Work out the finished part from the listing and answer in its coordinate system (mm). A direction names the side the tool comes from. Round coordinates to 2 decimals unless told otherwise and drop trailing zeros. Write each loop counter-clockwise with the first axis right and the second up, starting at its lowest first coordinate (ties: lowest second). Pieces come first, ordered by that corner, then holes.
1. Determine the mould class of faces 1 (the face through (-5.615, -25.284, 37.567)), 2 (the face through (3.175, 18, 32)), 3 (the face through (6.487, -20.284, 59.719)), 4 (the face through (0, -17, 0)) for opening direction X: pulls with the +X half, pulls with the -X half, needs draft (parallel to the pull), parting line crosses it, or undercut.
2. A tool of negligible diameter and unlimited length cuts with its end or side. For faces 5 (the face through (7.337, -14.106, 38.633)), 6 (the face through (0, 18, 35)), from which of +Z, -Z, +X, -X, +Y, -Y can it reach the whole face along a straight path? Write none if from no direction.
3. Find section A-A (y = 0). Write down the section's boundary in (x, z), and give its area (3 significant figures).
4. Find section C-C (x = -8.5). Write down the section's boundary in (y, z).
5. Straight lines are drawn through the part: probe 1 along Z at (x, y) = (0, 22); probe 2 along Y at (x, z) = (0, 18.5); probe 3 along Y at (x, z) = (0, 52). For each, find the intervals that lie inside material, in ascending order.
6. Flat-ended cylindrical pins translate along their axes: pin 1 Ø2 at (y, z) = (17.5, 13) entering from -X; pin 2 Ø2 at (y, z) = (-11.5, 9.5) entering from -X; pin 3 Ø4 at (x, z) = (12.5, 27) entering from +Y; pin 4 Ø5 at (y, z) = (0.5, 45) entering from -X. Find the tip coordinate at first contact, or state that the pin passes through.
7. Find section B-B (z = 8.5). Write down the section's boundary in (x, y) (3 decimals).
8. Find section D-D (x = 0). Count the separate pieces of the cut face and the enclosed holes in it, and give its area (3 significant figures).
```python
from build123d import *

# Parameters (mm, degrees)
SKETCH1_R                        = 25.9
BOSS_EXTRUDE1_DEPTH              = 76.2
SKETCH2_R                        = 15.9
CUT_EXTRUDE1_DEPTH               = 77.2
F_10_5_10_5_DIAMETER_HOLE1_D     = 10.5
F_10_5_10_5_DIAMETER_HOLE1_DEPTH = 20
F_10_5_10_5_DIAMETER_HOLE1_TIP   = 3.15451825
F_12_8_12_8_DIAMETER_HOLE1_D     = 12.8
F_12_8_12_8_DIAMETER_HOLE1_DEPTH = 300
F_12_8_12_8_DIAMETER_HOLE1_TIP   = 3.845507962
CUT_EXTRUDE2_DEPTH               = 35


with BuildPart() as part:
    # Sketch1 → Boss-Extrude1 (new body)
    with BuildSketch(Plane.XY):
        Circle(SKETCH1_R)
    extrude(amount=BOSS_EXTRUDE1_DEPTH)

    # Sketch2 → Cut-Extrude1 (cut, through all)
    with BuildSketch(Plane.XY.offset(76.2)):
        Circle(SKETCH2_R)
    extrude(amount=-CUT_EXTRUDE1_DEPTH, mode=Mode.SUBTRACT)

    # Ø10.5 (10.5) Diameter Hole1
    with Locations(Plane(origin=(0, 25.9, 25), x_dir=(0, 0, 1), z_dir=(0, 1, 0))):
        with Locations((0, 0)):
            Hole(F_10_5_10_5_DIAMETER_HOLE1_D / 2, depth=F_10_5_10_5_DIAMETER_HOLE1_DEPTH)
            with Locations((0, 0, -(F_10_5_10_5_DIAMETER_HOLE1_DEPTH + F_10_5_10_5_DIAMETER_HOLE1_TIP / 2))):  # 118° drill point
                Cone(0, F_10_5_10_5_DIAMETER_HOLE1_D / 2, F_10_5_10_5_DIAMETER_HOLE1_TIP, mode=Mode.SUBTRACT)

    # Ø12.8 (12.8) Diameter Hole1
    with Locations(Plane(origin=(-0.119429255, 25.899724644, 60), x_dir=(0.999989369, 0.004611168, 0), z_dir=(-0.004611168, 0.999989369, 0))):
        with Locations((0, 0)):
            Hole(F_12_8_12_8_DIAMETER_HOLE1_D / 2, depth=F_12_8_12_8_DIAMETER_HOLE1_DEPTH)
            with Locations((0, 0, -(F_12_8_12_8_DIAMETER_HOLE1_DEPTH + F_12_8_12_8_DIAMETER_HOLE1_TIP / 2))):  # 118° drill point
                Cone(0, F_12_8_12_8_DIAMETER_HOLE1_D / 2, F_12_8_12_8_DIAMETER_HOLE1_TIP, mode=Mode.SUBTRACT)

    # Sketch5 → Cut-Extrude2 (cut)
    with BuildSketch(Plane(origin=(0, 0, 0), x_dir=(-1, 0, 0), z_dir=(0, 0, -1))):
        with BuildLine():
            Line((-3.175, 20), (-3.175, 15.579774549))
            ThreePointArc((-3.175, 15.579774549), (0, 15.9), (3.175, 15.579774549))
            Line((3.175, 15.579774549), (3.175, 20))
            Line((3.175, 20), (-3.175, 20))
        make_face()
    extrude(amount=-CUT_EXTRUDE2_DEPTH, mode=Mode.SUBTRACT)


solid = part.part
```
Worked answers:
1. face 1: parting line crosses it
1. face 2: undercut
1. face 3: undercut
1. face 4: needs draft
2. face 5: +Z, -Z
2. face 6: -Z
3. outline: (-25.9, 0) - (-15.9, 0) - (-15.9, 76.2) - (-25.9, 76.2) - close; (15.9, 0) - (25.9, 0) - (25.9, 76.2) - (15.9, 76.2) - close
3. area: 1,520 mm2
4. outline: (-24.47, 0) - (-13.44, 0) - (-13.44, 76.2) - (-24.47, 76.2) - close; (13.44, 0) - (24.47, 0) - (24.47, 76.2) - (13.44, 76.2) - close
5. probe 1: z = 0 to 19.75, 30.25 to 53.6, 66.4 to 76.2
5. probe 2: y = -25.9 to -15.9, 20 to 25.9
5. probe 3: y = -25.9 to -15.9, 15.9 to 25.9
6. pin 1: stops at x = -19.96
6. pin 2: stops at x = -23.68
6. pin 3: stops at y = 23.68
6. pin 4: stops at x = -25.9
7. outline: circle Ø51.8 at (0, 0); hole (-3.175, 15.58) arc R15.9 ccw (long way) to (3.175, 15.58) - (3.175, 20) - (-3.175, 20) - close
8. separate pieces: 5
8. enclosed holes: 0
8. area: 1,060 mm2
